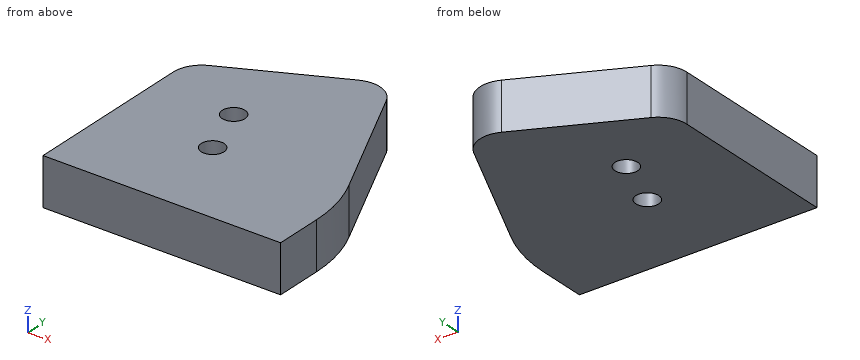
```python
from build123d import *

# Parameters (mm, degrees)
BOSS_EXTRUDE1_DEPTH  = 5
M2_CLEARANCE_HOLE1_D = 2.4
FILLET1_R            = 3


with BuildPart() as part:
    # Sketch1 → Boss-Extrude1 (new body)
    with BuildSketch(Plane.XY):
        with BuildLine():
            Line((-12.5, 17.5), (-12.5, -2.5))
            Line((-12.5, -2.5), (12.5, -2.5))
            Line((12.5, -2.5), (12.5, 2.5))
            ThreePointArc((12.5, 2.5), (12.144440107, 5.746594209), (11.094616806, 8.839273926))
            Line((11.094616806, 8.839273926), (4.755342879, 22.433890732))
            ThreePointArc((4.755342879, 22.433890732), (3.045285311, 23.991312891), (0.735528696, 23.869308605))
            Line((0.735528696, 23.869308605), (-12.5, 17.5))
        make_face()
    extrude(amount=BOSS_EXTRUDE1_DEPTH)

    # M2 Clearance Hole1 (through all)
    with Locations(Plane.XY.offset(5)):
        with Locations((-4.02606043, 12.819077862), (-1.97393957, 7.180922138)):
            Hole(M2_CLEARANCE_HOLE1_D / 2)

    # Fillet1
    fillet1_edges = [part.edges().sort_by_distance(p)[0] for p in [
        (-12.5, 17.5, 2.5),
    ]]
    fillet(fillet1_edges, radius=FILLET1_R)


solid = part.part
```
CAD build for the part. Positions are in the model's coordinates, mm. Round coordinates to 2 decimals unless told otherwise and drop trailing zeros. Order: outer loops, then holes, each group sorted by start corner. A loop starts at its lowest first (then second) coordinate and runs counter-clockwise, first axis right, second up. Notation, with made-up numbers: (14.25, -10) -> (71.25, -10) arc R19 ccw to (71.25, 1) -> close; hole circle Ø8 at (77.25, -1.75). An arc over 180 degrees is marked (long way). Write item = value, one per line.
(1) Cut at B-B (z = 3.6). Write the cut outline in (x, y), plus the area to 3 significant figures.
Answers follow:
outline = (-12.5, -2.5) -> (12.5, -2.5) -> (12.5, 2.5) arc R15 ccw to (11.09, 8.84) -> (4.76, 22.43) arc R3 ccw to (0.74, 23.87) -> (-10.8, 18.32) arc R3 ccw to (-12.5, 15.61) -> close; hole circle Ø2.4 at (-4.03, 12.82); hole circle Ø2.4 at (-1.97, 7.18)
area = 531 mm²
(2) Cut at D-D (y = 17.75). Write the cut outline in (x, z), plus the area to 3 significant figures.
Answers follow:
outline = (-11.61, 0) -> (6.94, 0) -> (6.94, 5) -> (-11.61, 5) -> close
area = 92.7 mm²
(3) Flat gauge pin, fed straight in: P1, Ø1.9, axis at x = -1.97, y = 7.18, coming from the +Z side. Where does the tip first touch, or does it go through?
Answers follow:
P1 = through
(4) Cut at A-A (y = 7.75). Write the cut outline in (x, z), plus the area to 3 significant figures.
Answers follow:
outline = (-12.5, 0) -> (-3.03, 0) -> (-3.03, 5) -> (-12.5, 5) -> close; (-0.92, 0) -> (11.55, 0) -> (11.55, 5) -> (-0.92, 5) -> close
area = 110 mm²
(5) Drill centre lines: L1, parallel to Y at x = -3.25, z = 0.65; L2, parallel to X at y = 6.75, z = 0.3; L3, parallel to Y at x = -4.75, z = 1.55. Where is each one in solid material? Low to high.
Answers follow:
L1 = -2.5 to 11.9, 13.73 to 21.95
L2 = -12.5 to -3.09, -0.85 to 11.89
L3 = -2.5 to 11.86, 13.78 to 21.23
(6) Cut at C-C (x = -3.75). Write the cut outline in (y, z), plus the area to 3 significant figures.
Answers follow:
outline = (-2.5, 0) -> (11.65, 0) -> (11.65, 5) -> (-2.5, 5) -> close; (13.99, 0) -> (21.71, 0) -> (21.71, 5) -> (13.99, 5) -> close
area = 109 mm²
